Check sheet for the drawn part. Datum: minimum x, y, z corner. Units: mm. A direction names the side the tool comes from. Round coordinates to 2 decimals unless told otherwise and drop trailing zeros. Order: outer loops, then holes, each group sorted by start corner. A loop starts at its lowest first (then second) coordinate and runs counter-clockwise, first axis right, second up. Notation, with made-up numbers: (75, 55) -> (95, 55) arc R5 ccw to (95, 61) -> close; hole circle Ø3 at (22.5, -35.5). An arc over 180 degrees is marked (long way). Write item = value, one per line. Start each with the question number.
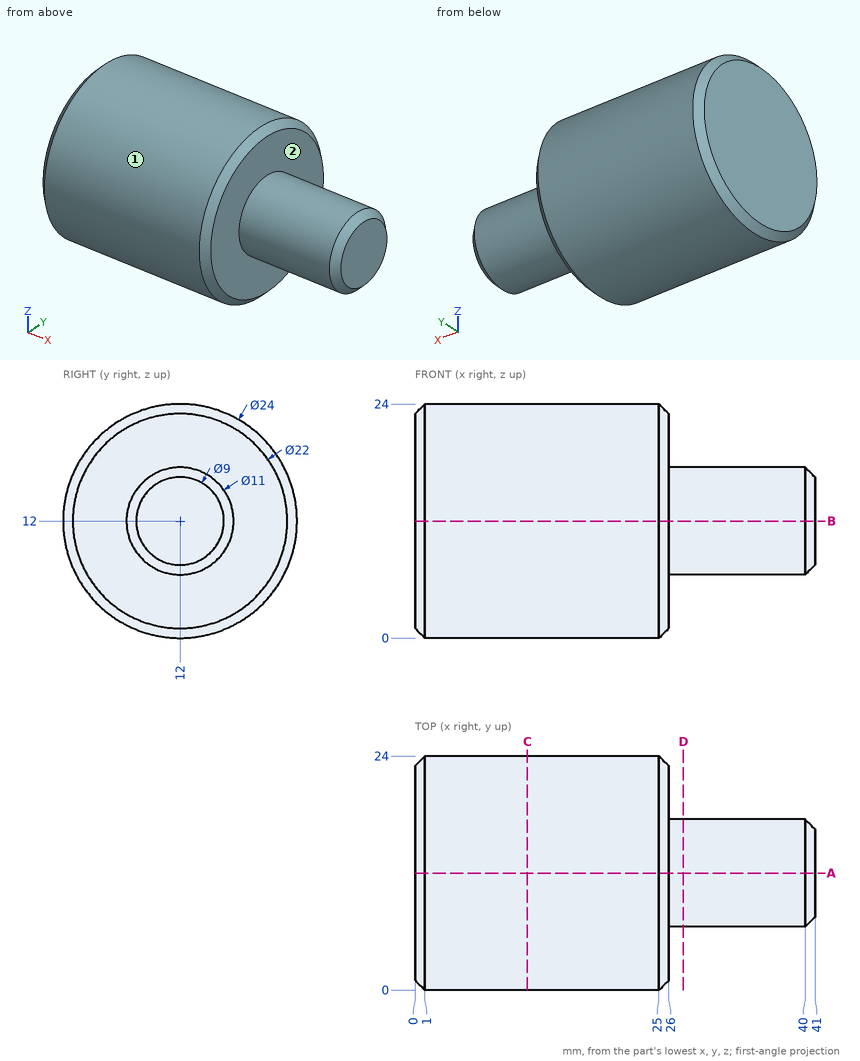
(1) Scan lines: line 1 along X through (y, z) = (6, 3.25); line 2 along X through (y, z) = (7.5, 22.5); line 3 along Y through (x, z) = (14.5, 22). Record each from-to range of solid material in increasing order. Write a range as from..to.
(2) Cross-section at D-D (x = 27.5). Enter the section's corners in (y, z).
(3) Set-up check for the marked faces 1 and 2: record each of +Z, -Z, +X, -X, +Y, -Y from which the full face is reachable in a straight line by a thin tool's end or side.
(4) Cross-section at A-A (y = 12). Enter the section's corners in (x, z).
(5) Cross-section at C-C (x = 11.5). Enter the section's corners in (y, z).
(6) Depth check by flat-ended pin: pin 1 (4 mm diameter, centred on y = 5.5, z = 3.5, fed in from -X); pin 2 (2 mm diameter, centred on x = 13, y = 16.5, fed in from -Z); pin 3 (5 mm diameter, centred on x = 32, z = 13, fed in from +Y); pin 4 (1 mm diameter, centred on x = 8.5, z = 18, fed in from +Y). Enter the tip coordinate at first touch or a pass-through.
Outcome:
q1.line_1 = 0..26
q1.line_2 = 0.42..25.58
q1.line_3 = 5.37..18.63
q2.outline = circle Ø11 at (12, 12)
q3.face_1 = +X, -X
q3.face_2 = +X
q4.outline = (0, 1) -> (1, 0) -> (25, 0) -> (26, 1) -> (26, 6.5) -> (40, 6.5) -> (41, 7.5) -> (41, 16.5) -> (40, 17.5) -> (26, 17.5) -> (26, 23) -> (25, 24) -> (1, 24) -> (0, 23) -> close
q5.outline = circle Ø24 at (12, 12)
q6.pin_1 = 0
q6.pin_2 = 0.52
q6.pin_3 = 17.5
q6.pin_4 = 22.67
